Geometry: final body of the model. Coordinates: model frame, mm. Face numbers are marked on the shaded views. A direction names the side the tool comes from. Round coordinates to 2 decimals unless told otherwise and drop trailing zeros. Loops run counter-clockwise (first coordinate to the right, second up) from the corner with the lowest first, then second, coordinate; pieces in that order, holes last. Notation, with made-up numbers: (42.5, 54.5) - (70.5, 54.5) arc R29 cw to (70.5, 76.5) - close; hole circle Ø9 at (55.25, 11.25). An arc over 180 degrees is marked (long way). Use CSV: the item, a comma, the result in double quotes.
from build123d import *

# Parameters (mm, degrees)
SKETCH1_R           = 12
SKETCH1_R_2         = 3.1
BOSS_EXTRUDE1_DEPTH = 10
CUT_EXTRUDE1_DEPTH  = 8
CHAMFER1_SIZE       = 1
CHAMFER1_SIZE2      = 1.732050808


with BuildPart() as part:
    # Sketch1 → Boss-Extrude1 (new body)
    with BuildSketch(Plane(origin=(0, 0, 0), x_dir=(1, 0, 0), z_dir=(0, 1, 0))):
        with Locations(Location((0, 0, 0), (0, 0, 270))):
            Circle(SKETCH1_R)
        with Locations(Location((0, 0, 0), (0, 0, 270))):
            Circle(SKETCH1_R_2, mode=Mode.SUBTRACT)
    extrude(amount=BOSS_EXTRUDE1_DEPTH)

    # Sketch2 → Cut-Extrude1 (cut)
    with BuildSketch(Plane(origin=(0, 10, 0), x_dir=(1, 0, 0), z_dir=(0, 1, 0))):
        Polygon((7.332348419, 0), (3.666174209, 6.35), (-3.666174209, 6.35), (-7.332348419, 0), (-3.666174209, -6.35), (3.666174209, -6.35), align=None)
    extrude(amount=-CUT_EXTRUDE1_DEPTH, mode=Mode.SUBTRACT)

    # Chamfer1
    chamfer1_edges = [part.edges().sort_by_distance(p)[0] for p in [
        (0, 0, -12),
    ]]
    chamfer1_side = [part.faces().sort_by_distance(p)[0] for p in [
        (0, 0, -11.660588745),
    ]]
    chamfer(chamfer1_edges, length=CHAMFER1_SIZE, length2=CHAMFER1_SIZE2, reference=chamfer1_side[0])


solid = part.part
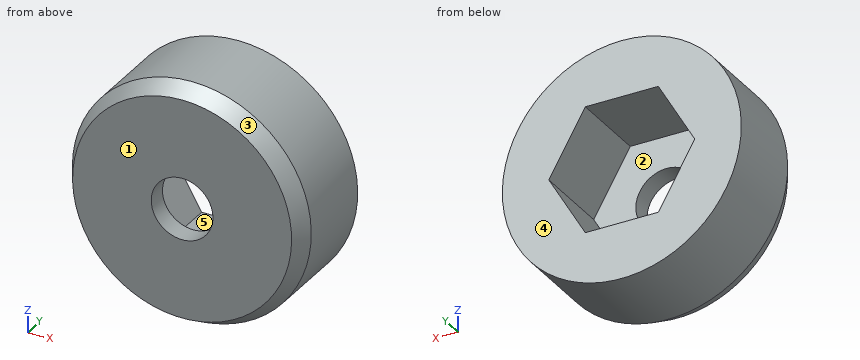
Item 1: Material intervals for line 1 (Z direction, x = -0.25, y = 6); line 2 (Y direction, x = 0.75, z = -6); line 3 (X direction, y = 6.75, z = -5.5), sorted ascending.
Final values:
line 1,"z = -12 to -6.35, 6.35 to 12"
line 2,"y = 0 to 2"
line 3,"x = -10.67 to -4.16, 4.16 to 10.67"
Item 2: Section B-B on y = 9.25. Return the cut outline in (x, z).
Final values:
outline,"circle Ø24 at (0, 0); hole (-7.33, 0) - (-3.67, -6.35) - (3.67, -6.35) - (7.33, 0) - (3.67, 6.35) - (-3.67, 6.35) - close"
Item 3: Pin query (flat end, axial travel): P1, Ø7, axis at x = 0, z = 0, coming from the -Y side; P2, Ø3, axis at x = -5.5, y = 2.5, coming from the -Z side; P3, Ø4, axis at x = -1.5, z = -2, coming from the +Y side; P4, Ø4, axis at y = 1, z = 8.5, coming from the +X side. Return the tip coordinate at first contact, or that it passes through.
Final values:
P1,"stops at y = 0"
P2,"stops at z = -11.31"
P3,"stops at y = 2"
P4,"stops at x = 10"
Item 4: Mould query, pull axis X, two halves, no side actions, for the marked faces 1, 2 and 3. Classes: released by +X, released by -X, zero draft, split by the parting line, or undercut.
Final values:
face 1,"zero draft"
face 2,"undercut"
face 3,"split by the parting line"
Item 5: Section A-A on x = 0. Return the cut outline in (y, z), plus the area to 3 significant figures.
Final values:
outline,"(0, -11) - (1.73, -12) - (10, -12) - (10, -6.35) - (2, -6.35) - (2, -3.1) - (0, -3.1) - close; (0, 3.1) - (2, 3.1) - (2, 6.35) - (10, 6.35) - (10, 12) - (1.73, 12) - (0, 11) - close"
area,"124 mm²"
Item 6: Reachability of the marked faces 4 and 5 from +Z, -Z, +X, -X, +Y, -Y: full face, straight path, thin tool, end or side. Return the list, or none.
Final values:
face 4,"+Z, -Z, +X, -X, +Y"
face 5,"+Y"
Item 7: Section C-C on y = 1. Return the cut outline in (x, z).
Final values:
outline,"circle Ø23.15 at (0, 0); hole circle Ø6.2 at (0, 0)"
